from build123d import *

# Parameters (mm, degrees)
SKETCH5_R           = 0.396875
BOSS_EXTRUDE2_DEPTH = 6.35
SKETCH6_R           = 2.9972
CUT_EXTRUDE1_DEPTH  = 258.501368276
SKETCH7_R           = 4.0005
CUT_EXTRUDE2_DEPTH  = 258.501368276


with BuildPart() as part:
    # Sketch5 → Boss-Extrude2 (new body)
    with BuildSketch(Plane(origin=(0, 0, 46.616707813), x_dir=(-1, 0, 0), z_dir=(0, 0, -1))):
        with BuildLine():
            ThreePointArc((246.921074011, -32.476835359), (246.808601397, -30.573015348), (246.075978074, -28.812207638))
            ThreePointArc((246.075978074, -28.812207638), (246.731600791, -28.342840277), (247.355067366, -27.831531862))
            ThreePointArc((247.355067366, -27.831531862), (248.865338892, -28.996117901), (250.674701217, -29.598935203))
            ThreePointArc((250.674701217, -29.598935203), (250.946601365, -29.309785139), (251.211187708, -29.013927881))
            ThreePointArc((251.211187708, -29.013927881), (250.454353229, -27.263390165), (249.163680793, -25.859344087))
            ThreePointArc((249.163680793, -25.859344087), (249.61923153, -25.194046866), (250.030220693, -24.500335994))
            ThreePointArc((250.030220693, -24.500335994), (251.847723585, -25.078145617), (253.754143671, -25.025770226))
            ThreePointArc((253.754143671, -25.025770226), (253.910751087, -24.661062717), (254.058191779, -24.292553976))
            ThreePointArc((254.058191779, -24.292553976), (252.748280843, -22.906439239), (251.055233439, -22.028503472))
            ThreePointArc((251.055233439, -22.028503472), (251.255766054, -21.247521054), (251.404706445, -20.455079495))
            ThreePointArc((251.404706445, -20.455079495), (253.310223032, -20.376420334), (255.083758479, -19.675169494))
            ThreePointArc((255.083758479, -19.675169494), (255.106183999, -19.278893649), (255.118695516, -18.882181018))
            ThreePointArc((255.118695516, -18.882181018), (253.413702715, -18.027675153), (251.522486845, -17.781741707))
            ThreePointArc((251.522486845, -17.781741707), (251.443814146, -16.979272099), (251.312741357, -16.183679999))
            ThreePointArc((251.312741357, -16.183679999), (253.076438214, -15.45803951), (254.503174475, -14.192494423))
            ThreePointArc((254.503174475, -14.192494423), (254.388713248, -13.812446955), (254.264786518, -13.435379832))
            ThreePointArc((254.264786518, -13.435379832), (252.370359146, -13.215548859), (250.509083356, -13.631280938))
            ThreePointArc((250.509083356, -13.631280938), (250.16069443, -12.904113816), (249.765417774, -12.201331325))
            ThreePointArc((249.765417774, -12.201331325), (251.174567032, -10.91623246), (252.082418656, -9.23903654))
            ThreePointArc((252.082418656, -9.23903654), (251.844876396, -8.921056785), (251.599458811, -8.60911503))
            ThreePointArc((251.599458811, -8.60911503), (249.744092768, -9.050473808), (248.137254388, -10.077727986))
            ThreePointArc((248.137254388, -10.077727986), (247.561170083, -9.513570439), (246.949365757, -8.988363496))
            ThreePointArc((246.949365757, -8.988363496), (247.834003218, -7.298808145), (248.113469901, -5.412255973))
            ThreePointArc((248.113469901, -5.412255973), (247.781497711, -5.19469698), (247.444190253, -4.985505373))
            ThreePointArc((247.444190253, -4.985505373), (245.851670066, -6.03481952), (244.69307752, -7.549693784))
            ThreePointArc((244.69307752, -7.549693784), (243.958782103, -7.216591536), (243.204242739, -6.932307851))
            ThreePointArc((243.204242739, -6.932307851), (243.457668071, -5.042081324), (243.075042005, -3.173718934))
            ThreePointArc((243.075042005, -3.173718934), (242.688680631, -3.08282153), (242.300167558, -3.001611666))
            ThreePointArc((242.300167558, -3.001611666), (241.162574665, -4.532318409), (240.591971311, -6.352096565))
            ThreePointArc((240.591971311, -6.352096565), (239.788031649, -6.290226665), (238.981765829, -6.281155045))
            ThreePointArc((238.981765829, -6.281155045), (238.573412195, -4.418246557), (237.574843733, -2.793426028))
            ThreePointArc((237.574843733, -2.793426028), (237.180694057, -2.840153782), (236.78783578, -2.896720768))
            ThreePointArc((236.78783578, -2.896720768), (236.242380673, -4.724194283), (236.328589698, -6.629384229))
            ThreePointArc((236.328589698, -6.629384229), (235.551972777, -6.846209099), (234.79122806, -7.113443716))
            ThreePointArc((234.79122806, -7.113443716), (233.770348935, -5.502547525), (232.27628017, -4.317246193))
            ThreePointArc((232.27628017, -4.317246193), (231.921882461, -4.495963046), (231.572063485, -4.68348407))
            ThreePointArc((231.572063485, -4.68348407), (231.6845361, -6.587304081), (232.417159423, -8.348111791))
            ThreePointArc((232.417159423, -8.348111791), (231.761536706, -8.817479152), (231.138070131, -9.328787567))
            ThreePointArc((231.138070131, -9.328787567), (229.627798605, -8.164201528), (227.818436279, -7.561384226))
            ThreePointArc((227.818436279, -7.561384226), (227.546536131, -7.850534289), (227.281949789, -8.146391548))
            ThreePointArc((227.281949789, -8.146391548), (228.038784268, -9.896929264), (229.329456703, -11.300975342))
            ThreePointArc((229.329456703, -11.300975342), (228.873905967, -11.966272563), (228.462916804, -12.659983435))
            ThreePointArc((228.462916804, -12.659983435), (226.645413911, -12.082173811), (224.738993826, -12.134549203))
            ThreePointArc((224.738993826, -12.134549203), (224.582386409, -12.499256711), (224.434945718, -12.867765452))
            ThreePointArc((224.434945718, -12.867765452), (225.744856653, -14.25388019), (227.437904058, -15.131815957))
            ThreePointArc((227.437904058, -15.131815957), (227.237371443, -15.912798374), (227.088431051, -16.705239934))
            ThreePointArc((227.088431051, -16.705239934), (225.182914465, -16.783899095), (223.409379017, -17.485149934))
            ThreePointArc((223.409379017, -17.485149934), (223.386953498, -17.88142578), (223.374441981, -18.278138411))
            ThreePointArc((223.374441981, -18.278138411), (225.079434782, -19.132644276), (226.970650651, -19.378577722))
            ThreePointArc((226.970650651, -19.378577722), (227.049323351, -20.18104733), (227.18039614, -20.97663943))
            ThreePointArc((227.18039614, -20.97663943), (225.416699282, -21.702279919), (223.989963022, -22.967825006))
            ThreePointArc((223.989963022, -22.967825006), (224.104424249, -23.347872473), (224.228350979, -23.724939596))
            ThreePointArc((224.228350979, -23.724939596), (226.122778351, -23.944770569), (227.98405414, -23.529038491))
            ThreePointArc((227.98405414, -23.529038491), (228.332443066, -24.256205612), (228.727719723, -24.958988104))
            ThreePointArc((228.727719723, -24.958988104), (227.318570464, -26.244086969), (226.410718841, -27.921282889))
            ThreePointArc((226.410718841, -27.921282889), (226.6482611, -28.239262644), (226.893678686, -28.551204399))
            ThreePointArc((226.893678686, -28.551204399), (228.749044729, -28.109845621), (230.355883108, -27.082591442))
            ThreePointArc((230.355883108, -27.082591442), (230.931967414, -27.64674899), (231.54377174, -28.171955932))
            ThreePointArc((231.54377174, -28.171955932), (230.659134278, -29.861511284), (230.379667596, -31.748063456))
            ThreePointArc((230.379667596, -31.748063456), (230.711639785, -31.965622448), (231.048947243, -32.174814056))
            ThreePointArc((231.048947243, -32.174814056), (232.64146743, -31.125499909), (233.800059977, -29.610625645))
            ThreePointArc((233.800059977, -29.610625645), (234.534355393, -29.943727892), (235.288894757, -30.228011577))
            ThreePointArc((235.288894757, -30.228011577), (235.035469426, -32.118238105), (235.418095491, -33.986600495))
            ThreePointArc((235.418095491, -33.986600495), (235.804456866, -34.077497898), (236.192969938, -34.158707763))
            ThreePointArc((236.192969938, -34.158707763), (237.330562832, -32.62800102), (237.901166185, -30.808222864))
            ThreePointArc((237.901166185, -30.808222864), (238.705105848, -30.870092764), (239.511371667, -30.879164384))
            ThreePointArc((239.511371667, -30.879164384), (239.919725301, -32.742072872), (240.918293764, -34.3668934))
            ThreePointArc((240.918293764, -34.3668934), (241.312443439, -34.320165647), (241.705301716, -34.263598661))
            ThreePointArc((241.705301716, -34.263598661), (242.250756824, -32.436125145), (242.164547799, -30.5309352))
            ThreePointArc((242.164547799, -30.5309352), (242.94116472, -30.31411033), (243.701909437, -30.046875713))
            ThreePointArc((243.701909437, -30.046875713), (244.722788562, -31.657771904), (246.216857327, -32.843073236))
            ThreePointArc((246.216857327, -32.843073236), (246.571255036, -32.664356383), (246.921074011, -32.476835359))
        make_face()
        with Locations((239.246568748, -18.580159714)):
            Circle(SKETCH5_R, mode=Mode.SUBTRACT)
    extrude(amount=-BOSS_EXTRUDE2_DEPTH)

    # Sketch6 → Cut-Extrude1 (cut, through all)
    with BuildSketch(Plane.XY.offset(52.966707813)):
        with Locations((-239.246568748, -18.580159714)):
            Circle(SKETCH6_R)
    extrude(amount=-CUT_EXTRUDE1_DEPTH, mode=Mode.SUBTRACT)

    # Sketch7 → Cut-Extrude2 (cut, through all)
    with BuildSketch(Plane.XY.offset(52.966707813)):
        with Locations((-239.246568748, -18.580159714)):
            Circle(SKETCH7_R)
    extrude(amount=-CUT_EXTRUDE2_DEPTH, mode=Mode.SUBTRACT)


solid = part.part
Can you work these out from the model? Positions are in its coordinate system, mm. A direction names the side the tool comes from. Round coordinates to 2 decimals unless told otherwise and drop trailing zeros. Loops run counter-clockwise (first coordinate to the right, second up) from the corner with the lowest first, then second, coordinate; pieces in that order, holes last. Notation, with made-up numbers: (-39, -12.5) - (-18, -12.5) arc R30 cw to (-18, 20.5) - close; hole circle Ø8 at (18.25, -18.75). An arc over 180 degrees is marked (long way). Use CSV: the item, a comma, the result in double quotes. Start each with the question number.
1) Please list where these lines run through material, in increasing order: probe 1 along X at (y, z) = (-5.5, 49.5); probe 2 along X at (y, z) = (-28, 51); probe 3 along Y at (x, z) = (-252.5, 52). Write a range as [from, to].
2) If we section it at A-A on x = -226: Write out the boundary of the cut face in (y, z), plus the area to 3 significant figures.
3) For pin 1 Ø2 at (y, z) = (-6.5, 48) entering from -X; pin 2 Ø1.5 at (x, z) = (-236, 48.5) entering from +Y (3 decimals); pin 3 Ø5 at (x, y) = (-239.25, -18.58) entering from +Z; pin 4 Ø1.5 at (y, z) = (-23, 48) entering from -X, each with a flat end and sliding along its axis, tell me the tip position at first contact or that it passes through.
4) For faces 1 (the cylindrical face through (-238.69, -30.87, 49.75)), 2 (the cylindrical face through (-250.47, -27.29, 49.75)), 3 (the cylindrical face through (-225.21, -16.78, 49.75)), 4 (the cylindrical face through (-227.048, -20.17, 49.747)), which set-ups out of +Z, -Z, +X, -X, +Y, -Y let a thin tool reach every point of the face, with its end or its side?
Geometry results:
1,probe 1,"x = [-248.11, -246.52], [-243.46, -240.78], [-238.89, -236.2], [-233.77, -231.54]"
1,probe 2,"x = [-250.86, -247.52], [-247.16, -231.33], [-228.99, -226.47]"
1,probe 3,"y = [-25.13, -22.73], [-20.49, -17.83], [-15.77, -13.21]"
2,outline,"(-23.95, 46.62) - (-21.38, 46.62) - (-21.38, 52.97) - (-23.95, 52.97) - close; (-19.33, 46.62) - (-16.67, 46.62) - (-16.67, 52.97) - (-19.33, 52.97) - close; (-14.44, 46.62) - (-12.03, 46.62) - (-12.03, 52.97) - (-14.44, 52.97) - close"
2,area,"48.5 mm2"
3,pin 1,"stops at x = -248.11"
3,pin 2,"stops at y = -2.975"
3,pin 3,"passes through"
3,pin 4,"stops at x = -253.65"
4,face 1,"+Z, -Z, -Y"
4,face 2,"+Z, -Z, -X"
4,face 3,"+Z, -Z"
4,face 4,"+Z, -Z, +X"
